Part print with two shaded views. Sizes in mm from the minimum x, y, z corner. Round coordinates to 2 decimals unless told otherwise and drop trailing zeros. Write each loop counter-clockwise with the first axis right and the second up, starting at its lowest first coordinate (ties: lowest second). Pieces come first, ordered by that corner, then holes. Notation, with made-up numbers: (87.5, 51.25) -> (129.5, 51.25) arc R35 cw to (129.5, 88.25) -> close; hole circle Ø9 at (45.5, -30). An arc over 180 degrees is marked (long way). Return JSON: item names as keys, results as strings.
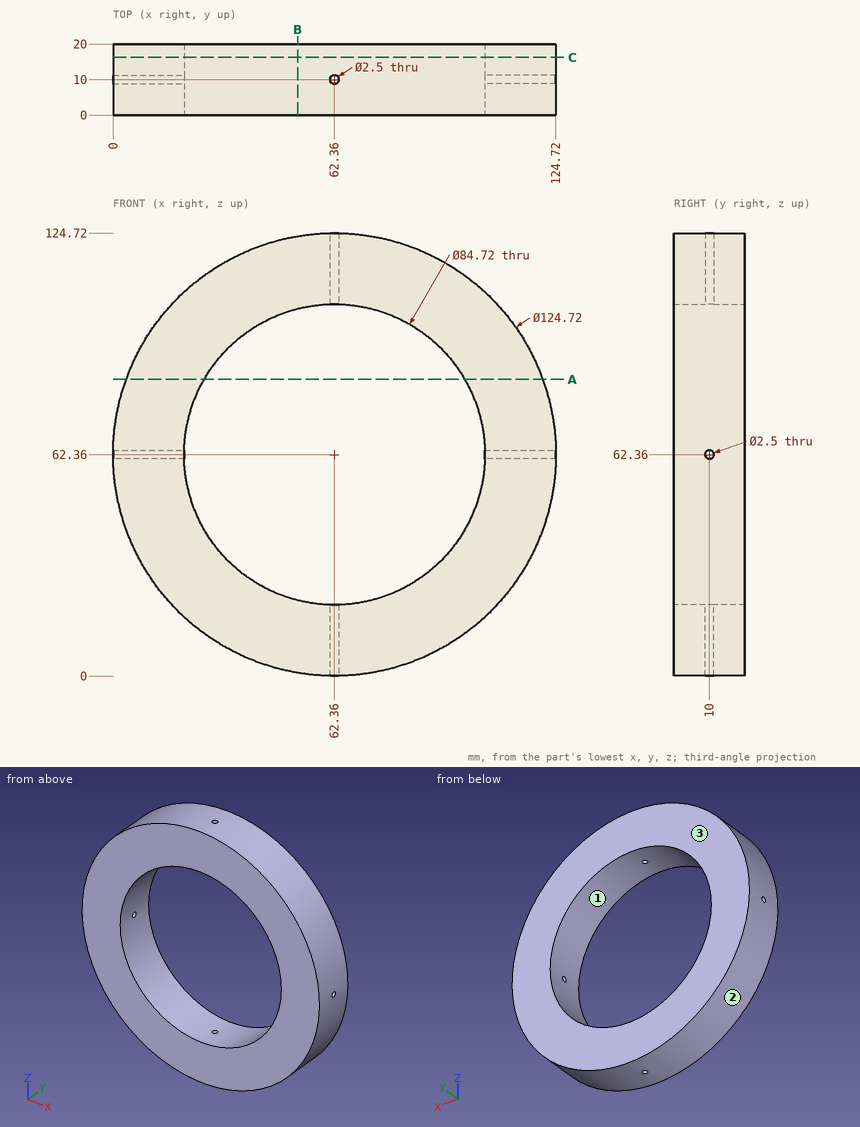
Q1. Saw through at B-B on x = 52. List the corners of the cut face in (y, z), then the cut area to 3 significant figures.
Verdict:
{"outline": "(0, 0.87) -> (20, 0.87) -> (20, 21.29) -> (0, 21.29) -> close; (0, 103.43) -> (20, 103.43) -> (20, 123.85) -> (0, 123.85) -> close", "area": "817 mm²"}
Q2. Wall check: L1, parallel to X at y = 7.25, z = 61; L2, parallel to Y at x = 8.25, z = 62.36. Give the ranges that are in metal, low to high.
Verdict:
{"L1": "x = 0.01 to 20.02, 104.7 to 124.71", "L2": "y = 0 to 8.75, 11.25 to 20"}
Q3. Saw through at A-A on z = 83.5. List the corners of the cut face in (x, y), then the cut area to 3 significant figures.
Verdict:
{"outline": "(3.69, 0) -> (25.65, 0) -> (25.65, 20) -> (3.69, 20) -> close; (99.07, 0) -> (121.03, 0) -> (121.03, 20) -> (99.07, 20) -> close", "area": "878 mm²"}
Q4. Two-plate mould, pull along Z, no slides. Class the marked faces 1, 2 and 3: +Z half, -Z half, draft (parallel to the pull), parting line (faces both ways), or undercut.
Verdict:
{"face 1": "undercut", "face 2": "parting line", "face 3": "draft"}
Q5. Saw through at C-C on y = 16.25. List the corners of the cut face in (x, z), then the cut area to 3 significant figures.
Verdict:
{"outline": "circle Ø124.72 at (62.36, 62.36); hole circle Ø84.72 at (62.36, 62.36)", "area": "6,580 mm²"}
Q6. Pin check, flat tips, straight feed: pin 1 Ø12 at (y, z) = (5.5, 53.5) entering from -X; pin 2 Ø2 at (y, z) = (18, 57.5) entering from +X; pin 3 Ø1 at (y, z) = (12, 17.5) entering from -X. Stop position of each tip, or through.
Verdict:
{"pin 1": "stops at x = 0.07", "pin 2": "stops at x = 124.6", "pin 3": "stops at x = 18.53"}
